Read the model definition and answer for the solid it produces. Units are mm, in the model's axes. Face numbers are marked on the shaded views. Give positions to 0.01 mm unless a question says otherwise; leave off trailing zeros. Order: outer loops, then holes, each group sorted by start corner. A loop starts at its lowest first (then second) coordinate and runs counter-clockwise, first axis right, second up.
```python
from build123d import *

# Parameters (mm, degrees)
F0_R     = 41.2696821878
F0_R_2   = 12.7004431624
F1_DEPTH = 9.525


# Not quite as in the source:
# - a feature names something its author has since deleted; it is built from what else it names


with BuildPart() as f1:
    # F0 (on Top) → F1 (new body)
    with BuildSketch(Plane.XY):
        Circle(F0_R)
        with BuildLine():
            ThreePointArc((34.593341478, 17.2228345975), (33.1984325721, 13.8552265986), (29.8308245732, 12.4603176927))
            Line((29.8308245732, 12.4603176927), (29.8308245732, -12.4556027445))
            ThreePointArc((29.8308245732, -12.4556027445), (33.201766544, -13.8518926268), (34.5980564262, -17.2228345975))
            ThreePointArc((34.5980564262, -17.2228345975), (31.0646749692, -21.8276269642), (25.7022806828, -19.606450524))
            Line((25.7022806828, -19.606450524), (4.1271236512, -32.062873244))
            ThreePointArc((4.1271236512, -32.062873244), (4.6032082956, -33.2122432496), (4.7655919019, -34.445669195))
            ThreePointArc((4.7655919019, -34.445669195), (-1.2334259454, -39.0488774906), (-4.1271236512, -32.062873244))
            Line((-4.1271236512, -32.062873244), (-25.7068508494, -19.6038119371))
            ThreePointArc((-25.7068508494, -19.6038119371), (-33.9547982971, -19.6038119371), (-29.8308245732, -12.4608799183))
            Line((-29.8308245732, -12.4608799183), (-29.8308245732, 12.464098707))
            ThreePointArc((-29.8308245732, 12.464098707), (-33.9520107443, 19.6022025428), (-25.7096384021, 19.6022025428))
            Line((-25.7096384021, 19.6022025428), (-4.1283119696, 32.062187168))
            ThreePointArc((-4.1283119696, 32.062187168), (-1.2337810845, 39.0502028877), (4.766964054, 34.445669195))
            ThreePointArc((4.766964054, 34.445669195), (4.6045336927, 33.2118881105), (4.1283119696, 32.062187168))
            Line((4.1283119696, 32.062187168), (25.7063639477, 19.6040930499))
            ThreePointArc((25.7063639477, 19.6040930499), (31.0634546508, 21.823072674), (34.593341478, 17.2228345975))
        make_face(mode=Mode.SUBTRACT)
        with BuildLine():
            Line((29.8308245732, -12.4556027445), (29.8308245732, 12.4603176927))
            ThreePointArc((29.8308245732, 12.4603176927), (25.7063639477, 14.8415761451), (25.7063639477, 19.6040930499))
            Line((25.7063639477, 19.6040930499), (4.1283119696, 32.062187168))
            ThreePointArc((4.1283119696, 32.062187168), (0, 29.6787051411), (-4.1283119696, 32.062187168))
            Line((-4.1283119696, 32.062187168), (-25.7096384021, 19.6022025428))
            ThreePointArc((-25.7096384021, 19.6022025428), (-25.2342386761, 18.4544860766), (-25.0720886827, 17.2228345975))
            ThreePointArc((-25.0720886827, 17.2228345975), (-26.4658901552, 13.8579001794), (-29.8308245732, 12.464098707))
            Line((-29.8308245732, 12.464098707), (-29.8308245732, -12.4608799183))
            ThreePointArc((-29.8308245732, -12.4608799183), (-26.4636141278, -13.8556241521), (-25.068869894, -17.2228345975))
            ThreePointArc((-25.068869894, -17.2228345975), (-25.231129565, -18.4553191604), (-25.7068508494, -19.6038119371))
            Line((-25.7068508494, -19.6038119371), (-4.1271236512, -32.062873244))
            ThreePointArc((-4.1271236512, -32.062873244), (0, -29.6800772931), (4.1271236512, -32.062873244))
            Line((4.1271236512, -32.062873244), (25.7022806828, -19.606450524))
            ThreePointArc((25.7022806828, -19.606450524), (25.7022806828, -14.839218671), (29.8308245732, -12.4556027445))
        make_face()
        Circle(F0_R_2, mode=Mode.SUBTRACT)
    extrude(amount=F1_DEPTH)


solid = f1.part
```
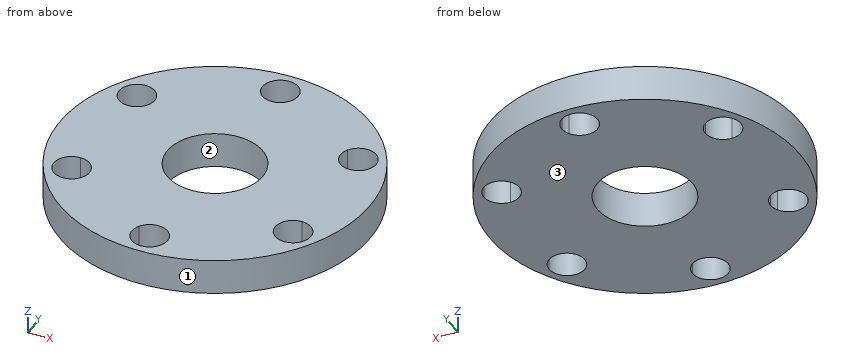
1) The part is cut by section D-D on y = -21. Determine the outline of the cut face in (x, z) (3 decimals).
Final values:
outline: (-35.527, 0) - (-32.731, 0) - (-32.731, 9.525) - (-35.527, 9.525) - close; (-26.931, 0) - (26.922, 0) - (26.922, 9.525) - (-26.931, 9.525) - close; (32.739, 0) - (35.527, 0) - (35.527, 9.525) - (32.739, 9.525) - close
2) The part is cut by section B-B on y = 0. Determine the outline of the cut face in (x, z) (3 decimals).
Final values:
outline: (-41.27, 0) - (-12.7, 0) - (-12.7, 9.525) - (-41.27, 9.525) - close; (12.7, 0) - (41.27, 0) - (41.27, 9.525) - (12.7, 9.525) - close
3) The part is cut by section C-C on z = 6.5. Determine the outline of the cut face in (x, y), and give its area (3 significant figures).
Final values:
outline: circle Ø82.54 at (0, 0); hole circle Ø9.52 at (-29.83, -17.22); hole circle Ø9.52 at (-29.83, 17.22); hole circle Ø25.4 at (0, 0); hole circle Ø9.53 at (0, -34.45); hole circle Ø9.53 at (0, 34.45); hole circle Ø9.53 at (29.83, -17.22); hole circle Ø9.53 at (29.83, 17.22)
area: 4,420 mm2
4) Given pin 1 (2 mm diameter, centred on y = 6.5, z = 5, fed in from -X); pin 2 (4 mm diameter, centred on x = -8, z = 5, fed in from +Y); pin 3 (4 mm diameter, centred on y = 13.5, z = 4.5, fed in from -X), each flat-ended and moving along its own axis, determine where each tip first touches the part or whether it passes through.
Final values:
pin 1: stops at x = -40.9
pin 2: stops at y = 40.83
pin 3: stops at x = -39.64
5) The part is cut by section A-A on x = 0. Determine the outline of the cut face in (y, z) (3 decimals).
Final values:
outline: (-41.27, 0) - (-39.211, 0) - (-39.211, 9.525) - (-41.27, 9.525) - close; (-29.68, 0) - (-12.7, 0) - (-12.7, 9.525) - (-29.68, 9.525) - close; (12.7, 0) - (29.679, 0) - (29.679, 9.525) - (12.7, 9.525) - close; (39.213, 0) - (41.27, 0) - (41.27, 9.525) - (39.213, 9.525) - close
6) Consider L1, parallel to X at y = -15.5, z = 6.5; L2, parallel to X at y = 21.5, z = 4.5; L3, parallel to X at y = 5, z = 7. Determine where each line is inside the solid, lowest interval first.
Final values:
L1: x = -38.25 to -34.27, -25.39 to 25.39, 34.28 to 38.25
L2: x = -35.23 to -31.92, -27.74 to 27.74, 31.93 to 35.23
L3: x = -40.97 to -11.67, 11.67 to 40.97
7) For a pull along Y with two mould halves and no side action, classify the marked faces 1, 2 and 3 as released by +Y, released by -Y, zero draft, split by the parting line, or undercut.
Final values:
face 1: split by the parting line
face 2: undercut
face 3: zero draft
